Check sheet for the modelled part. Datum: model origin and axes. Units: mm. Give positions to 0.01 mm unless a question says otherwise; leave off trailing zeros. Loops run counter-clockwise (first coordinate to the right, second up) from the corner with the lowest first, then second, coordinate; pieces in that order, holes last.
```python
from build123d import *

# Parameters (mm, degrees)
EXTRUDE_1_DEPTH = 5
SKETCH_2_R      = 2.5
EXTRUDE_2_DEPTH = 5


with BuildPart() as part:
    # 草图1 → 凸台-拉伸1 (new body)
    with BuildSketch(Plane(origin=(0, 0, 0), x_dir=(1, 0, 0), z_dir=(0, 1, 0))):
        with BuildLine():
            Line((0, 15), (30, 15))
            ThreePointArc((30, 15), (45, 0), (30, -15))
            Line((30, -15), (0, -15))
            ThreePointArc((0, -15), (-15, 0), (0, 15))
        make_face()
    extrude(amount=EXTRUDE_1_DEPTH)

    # 草图2 → 凸台-拉伸2 (add)
    with BuildSketch(Plane.XZ):
        with Locations(Location((0, 0, 0), (0, 0, 90))):
            Circle(SKETCH_2_R)
    extrude(amount=EXTRUDE_2_DEPTH)


solid = part.part
```
(1) Section check A-A on z = 0. Record the boundary of the cut face in (x, y), plus the area to 3 significant figures.
(2) Material ranges on line 1 (Y direction, x = -4, z = -11.5); line 2 (X direction, y = 3.25, z = 0.5); line 3 (X direction, y = 1.75, z = -5.5), recorded low to high.
(3) Section check C-C on x = 19. Record the boundary of the cut face in (y, z).
(4) Section check B-B on y = 4.25. Record the boundary of the cut face in (x, z).
(5) Gauge pin test, flat ends, axial feed: pin 1 Ø1.5 at (x, z) = (2, 5) entering from -Y; pin 2 Ø1.5 at (x, y) = (38, 0) entering from +Z; pin 3 Ø6 at (y, z) = (-1, 8.5) entering from +X; pin 4 Ø5 at (y, z) = (-3, -6) entering from +X. Record the tip position at first contact, or that the pin passes through.
(6) Release check for a two-part mould opening along X. For faces 1 (the face through (45, 2, 0)), 2 (the face through (2.44, -2.46, -0.54)), 3 (the face through (-15, 2, 0)), 4 (the face through (0, -5, 0)) record: pulls with the +X half, pulls with the -X half, needs draft (parallel to the pull), parting line crosses it, or undercut.
(7) Section check D-D on y = -3.5. Record the boundary of the cut face in (x, z), plus the area to 3 significant figures.
Computed values:
1. outline: (-15, 0) - (-2.5, 0) - (-2.5, -5) - (2.5, -5) - (2.5, 0) - (45, 0) - (45, 5) - (-15, 5) - close
1. area: 325 mm2
2. line 1: y = 0 to 5
2. line 2: x = -14.99 to 44.99
2. line 3: x = -13.96 to 43.96
3. outline: (0, -15) - (5, -15) - (5, 15) - (0, 15) - close
4. outline: (0, -15) - (30, -15) arc R15 ccw to (30, 15) - (0, 15) arc R15 ccw to start
5. pin 1: stops at y = 0
5. pin 2: stops at z = 13.13
5. pin 3: stops at x = 43.89
5. pin 4: passes through
6. face 1: pulls with the +X half
6. face 2: parting line crosses it
6. face 3: pulls with the -X half
6. face 4: needs draft
7. outline: circle Ø5 at (0, 0)
7. area: 19.6 mm2
